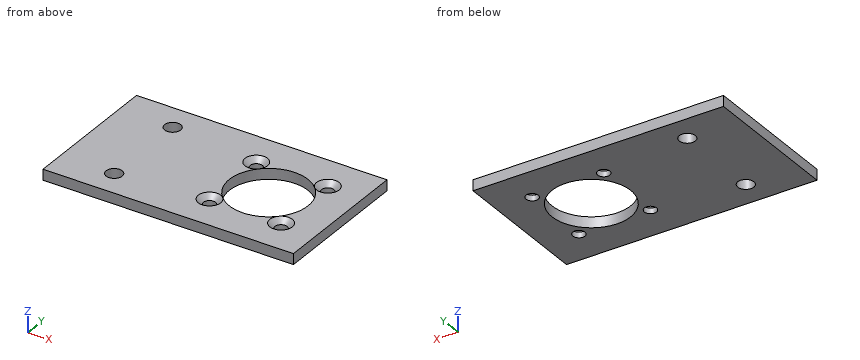
from build123d import *

# Parameters (mm, degrees)
SKIZZE1_W                                    = 70
SKIZZE1_H                                    = 40
AUFSATZ_LINEAR_AUSTRAGEN1_DEPTH              = 3
FORMSENKUNG_F_R_M3_LINSENSENKSCHRAUB_2_COUNT = 2
FORMSENKUNG_F_R_M3_LINSENSENKSCHRAUB_2_PITCH = 20
FORMSENKUNG_F_R_M3_LINSENSENKSCHRAUB_3_COUNT = 2
FORMSENKUNG_F_R_M3_LINSENSENKSCHRAUB_3_PITCH = 28.284271247
FORMSENKUNG_F_R_M3_LINSENSENKSCHRAUB_4_COUNT = 2
FORMSENKUNG_F_R_M3_LINSENSENKSCHRAUB_4_PITCH = 20
DURCHGANGSLOCH_F_R_M41_D                     = 4.5
F_22_0_22_DURCHMESSER_BOHRUNG1_D             = 22


with BuildPart() as part:
    # Skizze1 → Aufsatz-Linear austragen1 (new body)
    with BuildSketch(Plane.XY):
        with Locations((19.450005134, 330)):
            Rectangle(SKIZZE1_W, SKIZZE1_H)
    extrude(amount=AUFSATZ_LINEAR_AUSTRAGEN1_DEPTH)

    # Skizze3 → Formsenkung für M3 Linsensenkschraube mit Schlitz6 (revolve, cut)
    with BuildSketch(Plane(origin=(24.450005134, 340, 3), x_dir=(0, -1, 0), z_dir=(1, 0, 0))):
        Polygon((0, 0), (0, 3), (1.7, 3), (1.7, 1.45), (3.15, 0), align=None)
    formsenkung_f_r_m3_linsensenkschraube_mi = revolve(axis=Axis((24.450005134, 340, 9.35), (0, 0, -1)), mode=Mode.SUBTRACT)

    # Formsenkung f_r M3 Linsensenkschraub 2: Formsenkung für M3 Linsensenkschraube mit Schlitz6 ×2
    with Locations(*[(i * FORMSENKUNG_F_R_M3_LINSENSENKSCHRAUB_2_PITCH, 0, 0) for i in range(1, FORMSENKUNG_F_R_M3_LINSENSENKSCHRAUB_2_COUNT)]):
        add(formsenkung_f_r_m3_linsensenkschraube_mi, mode=Mode.SUBTRACT)

    # Formsenkung f_r M3 Linsensenkschraub 3: Formsenkung für M3 Linsensenkschraube mit Schlitz6 ×2
    with Locations(*[Vector(0.7071067811865485, -0.7071067811865466, 0) * (i * FORMSENKUNG_F_R_M3_LINSENSENKSCHRAUB_3_PITCH) for i in range(1, FORMSENKUNG_F_R_M3_LINSENSENKSCHRAUB_3_COUNT)]):
        add(formsenkung_f_r_m3_linsensenkschraube_mi, mode=Mode.SUBTRACT)

    # Formsenkung f_r M3 Linsensenkschraub 4: Formsenkung für M3 Linsensenkschraube mit Schlitz6 ×2
    with Locations(*[(0, -i * FORMSENKUNG_F_R_M3_LINSENSENKSCHRAUB_4_PITCH, 0) for i in range(1, FORMSENKUNG_F_R_M3_LINSENSENKSCHRAUB_4_COUNT)]):
        add(formsenkung_f_r_m3_linsensenkschraube_mi, mode=Mode.SUBTRACT)

    # Durchgangsloch für M41 (through all)
    with Locations(Plane.XY.offset(3)):
        with Locations((-0.549994866, 342.5), (-0.549994866, 317.5)):
            Hole(DURCHGANGSLOCH_F_R_M41_D / 2)

    # Ø22.0 (22) Durchmesser Bohrung1 (through all)
    with Locations(Plane(origin=(0, 0, 0), x_dir=(-1, 0, 0), z_dir=(0, 0, -1))):
        with Locations((-34.450005134, 330)):
            Hole(F_22_0_22_DURCHMESSER_BOHRUNG1_D / 2)


solid = part.part
Could you check a few things on this model? Use its own coordinates, in mm. Give positions to 0.01 mm unless a question says otherwise; leave off trailing zeros. Order: outer loops, then holes, each group sorted by start corner. A loop starts at its lowest first (then second) coordinate and runs counter-clockwise, first axis right, second up. Notation, with made-up numbers: (59.5, 88.25) -> (73.5, 88.25) arc R7 cw to (73.5, 99.25) -> close; hole circle Ø11 at (51.5, 15.25). An arc over 180 degrees is marked (long way). Answer in a Markdown table with one row per item. Add a question column.
Item 1: I'm going to push flat-ended pins straight in: P1, Ø2.5, axis at x = -0.55, y = 317.5, coming from the +Z side; P2, Ø4.5, axis at x = 44.45, y = 320, coming from the +Z side. Where does each tip first touch, or does it pass through?
Item 2: Imagine slicing it at A-A (y = 330). List the corners of the cut face in (x, z) for me.
Item 3: Please list where these lines run through material, in increasing order: probe 1 along Y at (x, z) = (43.5, 1.4); probe 2 along Y at (x, z) = (34.5, 2.15); probe 3 along Y at (x, z) = (23, 2.65).
Result:
| question | item | result |
|---|---|---|
| 1 | P1 | through |
| 1 | P2 | z = 2.1 |
| 2 | outline | (-15.55, 0) -> (23.45, 0) -> (23.45, 3) -> (-15.55, 3) -> close; (45.45, 0) -> (54.45, 0) -> (54.45, 3) -> (45.45, 3) -> close |
| 3 | probe 1 | 310 to 318.59, 321.41 to 323.75, 336.25 to 338.59, 341.41 to 350 |
| 3 | probe 2 | 310 to 319, 341 to 350 |
| 3 | probe 3 | 310 to 317.6, 322.4 to 337.6, 342.4 to 350 |
